For this review, take the finished solid that the model builds, in its own axes (mm). A direction names the side the tool comes from. Round coordinates to 2 decimals unless told otherwise and drop trailing zeros. Write each loop counter-clockwise with the first axis right and the second up, starting at its lowest first coordinate (ties: lowest second). Pieces come first, ordered by that corner, then holes. Notation, with made-up numbers: M 6.5,-1.5 L 18.5,-1.5 A9 ccw 18.5,8.5 Z; hole C 80.25,-22.5 d3. An arc over 180 degrees is marked long. One line per question, with ' | ' between items.
```python
from build123d import *

# Parameters (mm, degrees)
F0_W     = 150
F0_H     = 88.9
F0_W_2   = 100
F0_H_2   = 18.9
F1_DEPTH = 25
F2_DEPTH = 190


# Not quite as in the source:
# - an extrude ends at something that could not be found from the text; its depth is read off the source's solid


with BuildPart() as f1:
    # F0 (on Front) → F1 (new body)
    with BuildSketch(Plane.XZ):
        with Locations((3.1299684197, -4.7291009414)):
            Rectangle(F0_W, F0_H)
        with Locations((3.1299684197, -4.7291009414)):
            Rectangle(F0_W_2, F0_H_2, mode=Mode.SUBTRACT)
    extrude(amount=F1_DEPTH)

    # F0 (on Front) → F2 (cut, through all)
    with BuildSketch(Plane.XZ):
        with Locations((3.1299684197, -4.7291009414)):
            Rectangle(F0_W_2, F0_H_2)
    extrude(amount=-F2_DEPTH, mode=Mode.SUBTRACT)


solid = f1.part
```
Item 1: Take a section at B-B (x = 31). Write out the cut boundary in (y, z).
Results:
outline: M -25,-49.18 L 0,-49.18 L 0,-14.18 L -25,-14.18 Z; M -25,4.72 L 0,4.72 L 0,39.72 L -25,39.72 Z
Item 2: Mouldability with a two-part tool opening along Z and no side actions: class faces 3 (the face through (2, -12, 39.721)), 4 (the face through (53.13, -12, -5)), 5 (the face through (2, -12, -49.179)), 6 (the face through (78.13, -12, -5)) as +Z half, -Z half, draft (parallel to the pull), parting line (faces both ways), or undercut.
Results:
face 3: +Z half | face 4: undercut | face 5: -Z half | face 6: draft
Item 3: To check wall thickness, follow line 1 along Z through (x, y) = (32, -20.5); line 2 along X through (y, z) = (-6.5, -3). State the ranges of each line that lie inside material, in increasing order. Write a range as from..to.
Results:
line 1: -49.18..-14.18, 4.72..39.72 | line 2: -71.87..-46.87, 53.13..78.13
Item 4: Take a section at A-A (y = -5). Write out the cut boundary in (x, z).
Results:
outline: M -71.87,-49.18 L 78.13,-49.18 L 78.13,39.72 L -71.87,39.72 Z; hole M -46.87,-14.18 L 53.13,-14.18 L 53.13,4.72 L -46.87,4.72 Z
Item 5: Machinability: for faces 1 (the face through (-46.87, -12, -5)), 2 (the face through (2, -25, 6)), which of the approach directions +Z, -Z, +X, -X, +Y, -Y give a long, thin tool a straight path to every point of the face, cutting with its end or side? Answer none if there is none.
Results:
face 1: +Y, -Y | face 2: +Z, -Z, +X, -X, -Y
